Can you work these out from the model? Positions are in its coordinate system, mm. Face numbers are marked on the shaded views. A direction names the side the tool comes from. Give positions to 0.01 mm unless a question says otherwise; leave off trailing zeros. Write each loop counter-clockwise with the first axis right and the second up, starting at its lowest first coordinate (ties: lowest second). Pieces come first, ordered by that corner, then holes. Notation, with made-up numbers: M 39.5,78.25 L 54.5,78.25 A34 cw 54.5,111.25 Z; hole C -16.5,63.25 d4. An arc over 180 degrees is marked long. Write each question's results on one line, items separated by ' | '.
from build123d import *

# Parameters (mm, degrees)
F0_W     = 25.4
F0_H     = 9.525
F1_DEPTH = 4.699
F3_DEPTH = 3.175
F4_R     = 1.190625
F5_DEPTH = 9.399
F6_R     = 2.54


with BuildPart() as f1:
    # F0 (on Right) → F1 (new body, symmetric)
    with BuildSketch(Plane.YZ):
        with Locations((0, 4.7625)):
            Rectangle(F0_W, F0_H)
    extrude(amount=F1_DEPTH, both=True)

    # F2 (on Right) → F3 (join, symmetric)
    with BuildSketch(Plane.YZ):
        with BuildLine():
            Line((3.175, 17.4625), (5.715, 17.4625))
            ThreePointArc((5.715, 17.4625), (0, 23.1775), (-5.715, 17.4625))
            Line((-5.715, 17.4625), (-3.175, 17.4625))
            ThreePointArc((-3.175, 17.4625), (0, 20.6375), (3.175, 17.4625))
        make_face()
        with BuildLine():
            Line((5.715, 0), (5.715, 17.4625))
            ThreePointArc((5.715, 17.4625), (0, 11.7475), (-5.715, 17.4625))
            Line((-5.715, 17.4625), (-5.715, 0))
            Line((-5.715, 0), (5.715, 0))
        make_face()
        with BuildLine():
            ThreePointArc((-5.715, 17.4625), (0, 11.7475), (5.715, 17.4625))
            Line((5.715, 17.4625), (3.175, 17.4625))
            ThreePointArc((3.175, 17.4625), (0, 14.2875), (-3.175, 17.4625))
            Line((-3.175, 17.4625), (-5.715, 17.4625))
        make_face()
    extrude(amount=F3_DEPTH, both=True)

    # F4 (on face) → F5 (cut, through all)
    with BuildSketch(Plane.YZ.offset(4.699)):
        with Locations((-6.35, 4.7625)):
            Circle(F4_R)
        with Locations((6.35, 4.7625)):
            Circle(F4_R)
    extrude(amount=-F5_DEPTH, mode=Mode.SUBTRACT)

    # F6
    f6_edges = [f1.edges().sort_by_distance(p)[0] for p in [
        (0, 5.715, 9.525),
        (0, -5.715, 9.525),
    ]]
    fillet(f6_edges, radius=F6_R)


solid = f1.part
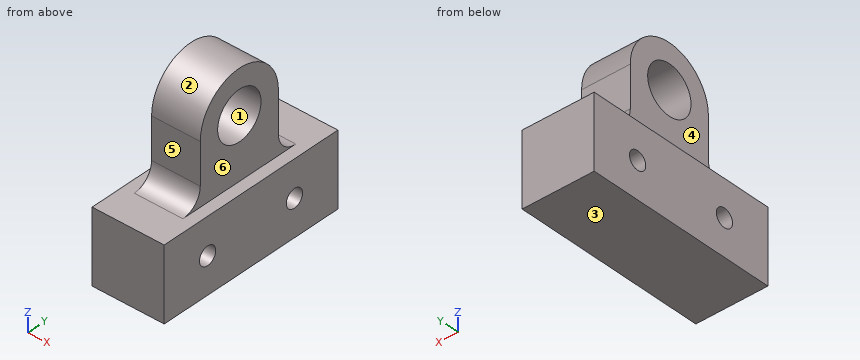
Item 1: I'm going to push flat-ended pins straight in: pin 1 (4 mm diameter, centred on y = 7, z = 17.5, fed in from -X) (3 decimals); pin 2 (3 mm diameter, centred on y = -0.5, z = 15, fed in from +X) (3 decimals); pin 3 (2.5 mm diameter, centred on x = -1.5, z = 15, fed in from -Y) (3 decimals); pin 4 (8 mm diameter, centred on y = -10, z = 20, fed in from -X). Where does each tip first touch, or does it pass through?
Geometry says:
pin 1: stops at x = -3.175 | pin 2: stops at x = 3.175 | pin 3: stops at y = -5.715 | pin 4: passes through
Item 2: Thinking about a two-plate mould opening in Y: for the marked faces 1, 2 and 3, which applies, +Y half, -Y half, draft (parallel to the pull), parting line (faces both ways), or undercut?
Geometry says:
face 1: undercut | face 2: parting line | face 3: draft
Item 3: I want a section at B-B, the plane z = 15. Please give me the cut outline in (x, y) (3 decimals).
Geometry says:
outline: M -3.175,-5.715 L 3.175,-5.715 L 3.175,-2.004 L -3.175,-2.004 Z; M -3.175,2.004 L 3.175,2.004 L 3.175,5.715 L -3.175,5.715 Z
Item 4: I want a section at A-A, the plane y = 0. Please give me the cut outline in (x, z) (1 decimal).
Geometry says:
outline: M -4.7,0 L 4.7,0 L 4.7,9.5 L 3.2,9.5 L 3.2,14.3 L -3.2,14.3 L -3.2,9.5 L -4.7,9.5 Z; M -3.2,20.6 L 3.2,20.6 L 3.2,23.2 L -3.2,23.2 Z
Item 5: For the marked faces 4, 5 and 6, which set-ups out of +Z, -Z, +X, -X, +Y, -Y let a thin tool reach every point of the face, with its end or its side?
Geometry says:
face 4: +Z, -X, +Y, -Y | face 5: +Z, +X, -X, -Y | face 6: +Z, +X, +Y, -Y
Item 6: If I drill on line 1 (Z direction, x = 1.5, y = 0); line 2 (Z direction, x = -2.25, y = 10.5) (3 decimals); line 3 (Z direction, x = 2.75, y = -6.35), over which ranges is the centre line in solid material (lowest first)? Write a range as from..to.
Geometry says:
line 1: z = 0..14.29, 20.64..23.18 | line 2: z = 0..9.525 | line 3: z = 0..3.57, 5.95..10.38
Item 7: I want a section at C-C, the plane x = -0.75. Give the number of separate pieces and of enclosed holes in the cut face, and give its area (3 significant figures).
Geometry says:
separate pieces: 1 | enclosed holes: 3 | area: 346 mm2
